Part print with two shaded views. Sizes in mm from the minimum x, y, z corner. A direction names the side the tool comes from. Coordinates: 2 decimals unless noted, no trailing zeros. Write each loop counter-clockwise with the first axis right and the second up, starting at its lowest first coordinate (ties: lowest second). Pieces come first, ordered by that corner, then holes. Notation, with made-up numbers: (-23.75, -34) - (-8.75, -34) arc R11 cw to (-8.75, -27) - close; hole circle Ø5 at (38.5, 21.5). An arc over 180 degrees is marked (long way). Answer in a Markdown table with one row per item. Add a question column.
Q1. Band-saw the part on D-D (x = 17). List the corners of the cut face in (y, z), and give its area (3 significant figures).
Q2. Band-saw the part on C-C (x = 23). List the corners of the cut face in (y, z).
Q3. Band-saw the part on A-A (z = 6.25). List the corners of the cut face in (x, y), and give its area (3 significant figures).
Q4. Drill centre lines: line 1 along Z through (x, y) = (18.75, 0.75); line 2 along Y through (x, z) = (16.75, 2.75); line 3 along Y through (x, z) = (5.25, 7). Where is each one in solid material? Low to high. Write a range as from..to.
Q5. Two-plate mould, pull along Y, no slides. Class the marked faces 1, 2 and 3: +Y half, -Y half, draft (parallel to the pull), parting line (faces both ways), or undercut.
Q6. Band-saw the part on B-B (y = 9). List the corners of the cut face in (x, z).
Q7. 3-axis set-ups, long thin cutter, end or side, ignore diameter. For the marked faces 4, 5 and 6: which of +Z, -Z, +X, -X, +Y, -Y reach the whole face in a straight line?
Q8. Pin check, flat tips, straight feed: pin 1 (4 mm diameter, centred on y = 11, z = 7, fed in from +X); pin 2 (4 mm diameter, centred on x = 18.75, z = 6.25, fed in from -Y); pin 3 (4 mm diameter, centred on x = 5, y = 9, fed in from -Z); pin 4 (10.5 mm diameter, centred on x = 6, y = 7, fed in from +Z). Stop position of each tip, or through.
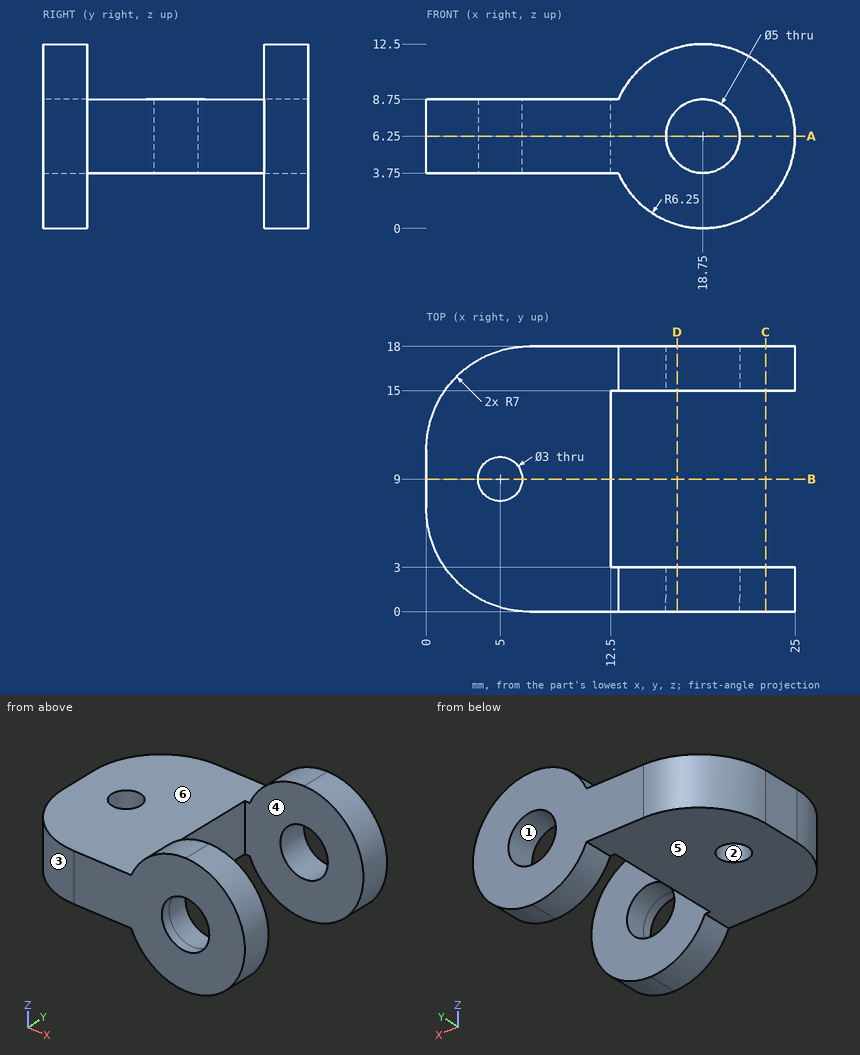
Checked values:
| question | item | result |
|---|---|---|
| 1 | outline | (0, 0.25) - (3, 0.25) - (3, 4.46) - (0, 4.46) - close; (0, 8.04) - (3, 8.04) - (3, 12.25) - (0, 12.25) - close; (15, 0.25) - (18, 0.25) - (18, 4.46) - (15, 4.46) - close; (15, 8.04) - (18, 8.04) - (18, 12.25) - (15, 12.25) - close |
| 1 | area | 50.6 mm² |
| 2 | outline | (0, 1.67) - (3, 1.67) - (3, 10.83) - (0, 10.83) - close; (15, 1.67) - (18, 1.67) - (18, 10.83) - (15, 10.83) - close |
| 3 | outline | (0, 7) arc R7 ccw to (7, 0) - (16.25, 0) - (16.25, 3) - (12.5, 3) - (12.5, 15) - (16.25, 15) - (16.25, 18) - (7, 18) arc R7 ccw to (0, 11) - close; (21.25, 0) - (25, 0) - (25, 3) - (21.25, 3) - close; (21.25, 15) - (25, 15) - (25, 18) - (21.25, 18) - close; hole circle Ø3 at (5, 9) |
| 3 | area | 242 mm² |
| 4 | line 1 | z = 0..3.75, 8.75..12.5 |
| 4 | line 2 | y = 0..3, 15..18 |
| 4 | line 3 | y = 0.22..7.52, 10.48..17.78 |
| 5 | face 1 | draft |
| 5 | face 2 | undercut |
| 5 | face 3 | -Y half |
| 6 | outline | (0, 3.75) - (3.5, 3.75) - (3.5, 8.75) - (0, 8.75) - close; (6.5, 3.75) - (12.5, 3.75) - (12.5, 8.75) - (6.5, 8.75) - close |
| 7 | face 4 | +Z, -Z, +X |
| 7 | face 5 | -Z, -X, +Y, -Y |
| 7 | face 6 | +Z, -X, +Y, -Y |
| 8 | pin 1 | stops at x = 12.5 |
| 8 | pin 2 | passes through |
| 8 | pin 3 | stops at z = 3.75 |
| 8 | pin 4 | stops at z = 8.75 |
